Solid Edge part; units mm, degrees
sketch "Sketch1" plane through (0, 0, 0) normal (0, 1, 0) x (-1, 0, 0)
  line L0 (-4.7625, -4.76) -> (4.7625, -4.76)
  line L1 (4.7625, -4.76) -> (4.7625, 4.76)
  line L2 (4.7625, 4.76) -> (-4.7625, 4.76)
  line L3 (-4.7625, 4.76) -> (-4.7625, -4.76)
extrude "Protrusion1" add sketch "Sketch1" along normal mid plane 15
sketch "Sketch2" plane through (0, 7.5, 0) normal (0, 1, 0) x (-1, 0, 0)
  circle A0 centre (0, 0) radius 3.175
extrude "Cutout1" cut sketch "Sketch2" against normal up to surface (15 mm away)
fillet "Round_1" radius 4.755 2 edges at (-4.7625, 0, 4.76) (4.7625, 0, 4.76)
Build history of the part. All positions in model axes, mm. Round coordinates to 2 decimals unless told otherwise and drop trailing zeros. Loops run counter-clockwise (first coordinate to the right, second up) from the corner with the lowest first, then second, coordinate; pieces in that order, holes last. Notation, with made-up numbers: (61, 62.25) -> (66, 62.25) arc R21 ccw to (66, 66.25) -> close; hole circle Ø9 at (21.25, 17.25). An arc over 180 degrees is marked (long way). One line per item, written item: value. Start each with the question number.
Q1. Cut at A-A on z = -0.5. List the corners of the cut face in (x, y).
Q2. Two-plate mould, pull along X, no slides. Class faces 1 (the face through (4.762, 0, -2)), 2 (the face through (-4.762, 0, -2)), 3 (the face through (0.69, 0.11, -3.1)), 4 (the face through (0, 0, -4.76)): released by +X, released by -X, zero draft, split by the parting line, or undercut.
Q3. Drop flat-ended pins along their axis: pin 1 Ø1 at (x, y) = (2.5, 2) entering from +Z; pin 2 Ø1 at (x, z) = (-1.5, 0.5) entering from +Y. Give the stop position or say it passes through.
Q4. Cut at B-B on x = -1. List the corners of the cut face in (y, z).
Q5. Cut at D-D on x = 3.75. List the corners of the cut face in (y, z).
Q6. Probe line 1 along Z through (x, y) = (0, 4.25) (3 decimals); line 2 along Z through (x, y) = (1.75, 1.5); line 3 along X through (y, z) = (-3, -0.75). List the from-to ranges inside material, lowest first.
Computed:
1. outline: (-4.76, -7.5) -> (-3.14, -7.5) -> (-3.14, 7.5) -> (-4.76, 7.5) -> close; (3.14, -7.5) -> (4.76, -7.5) -> (4.76, 7.5) -> (3.14, 7.5) -> close
2. face 1: released by +X
2. face 2: released by -X
2. face 3: undercut
2. face 4: zero draft
3. pin 1: z = 4.32
3. pin 2: through
4. outline: (-7.5, -4.76) -> (7.5, -4.76) -> (7.5, -3.01) -> (-7.5, -3.01) -> close; (-7.5, 3.01) -> (7.5, 3.01) -> (7.5, 4.66) -> (-7.5, 4.66) -> close
5. outline: (-7.5, -4.76) -> (7.5, -4.76) -> (7.5, 2.94) -> (-7.5, 2.94) -> close
6. line 1: -4.76 to -3.175, 3.175 to 4.76
6. line 2: -4.76 to -2.65, 2.65 to 4.43
6. line 3: -4.76 to -3.09, 3.09 to 4.76
